Geometry: final body of the model. Coordinates: model frame, mm. A direction names the side the tool comes from. Give positions to 0.01 mm unless a question says otherwise; leave off trailing zeros. Write each loop counter-clockwise with the first axis right and the second up, starting at its lowest first coordinate (ties: lowest second). Pieces come first, ordered by that corner, then holes.
```python
from build123d import *

# Parameters (mm, degrees)
SKETCH1_R               = 8.25
BOSS_EXTRUDE1_DEPTH     = 135
BOSS_EXTRUDE2_DEPTH     = 2
CUT_EXTRUDE1_DEPTH      = 138.727992797
CUT_EXTRUDE1_DEPTH_BACK = 138.727992797
SKETCH4_R               = 1.6
SKETCH4_R_2             = 2.6
SKETCH4_R_3             = 3.727922061
SKETCH6_R               = 1.4
CUT_EXTRUDE2_DEPTH      = 140.11090078
CIRPATTERN1_COUNT       = 2
CIRPATTERN1_ANGLE       = 270
SKETCH7_R               = 6.269832862
CUT_EXTRUDE3_DEPTH      = 138.727992904


with BuildPart() as part:
    # Sketch1 → Boss-Extrude1 (new body)
    with BuildSketch(Plane.XY):
        Polygon((10, 4.142135624), (4.142135624, 10), (-4.142135624, 10), (-10, 4.142135624), (-10, -4.142135624), (-4.142135624, -10), (4.142135624, -10), (10, -4.142135624), align=None)
        Circle(SKETCH1_R, mode=Mode.SUBTRACT)
    extrude(amount=-BOSS_EXTRUDE1_DEPTH)

    # Sketch2 → Boss-Extrude2 (add)
    with BuildSketch(Plane(origin=(0, 0, -135), x_dir=(-1, 0, 0), z_dir=(0, 0, -1))):
        Polygon((-10, 4.142135624), (-10, -4.142135624), (-4.142135624, -10), (4.142135624, -10), (10, -4.142135624), (10, 4.142135624), (4.142135624, 10), (-4.142135624, 10), align=None)
    extrude(amount=BOSS_EXTRUDE2_DEPTH)

    # Sketch4 → Cut-Extrude1 (cut, two sides: drawn at the far end of the back side and taken through both)
    with BuildSketch(Plane(origin=(0, 0, 0), x_dir=(1, 0, 0), z_dir=(0, 1, 0)).offset(-CUT_EXTRUDE1_DEPTH_BACK)):
        with Locations(Location((0, 131.593089119, 0), (0, 0, 270))):
            Circle(SKETCH4_R)
        with Locations(Location((0, 106.593089119, 0), (0, 0, 270))):
            Circle(SKETCH4_R)
        with Locations(Location((0, 35, 0), (0, 0, 270))):
            Circle(SKETCH4_R_2)
        with Locations(Location((0, 119.093089119, 0), (0, 0, 270))):
            Circle(SKETCH4_R_3)
    extrude(amount=CUT_EXTRUDE1_DEPTH + CUT_EXTRUDE1_DEPTH_BACK, mode=Mode.SUBTRACT)

    # Sketch6 → Cut-Extrude2 (cut, through all)
    with BuildSketch(Plane(origin=(-7.071067812, 7.071067812, 0), x_dir=(0, 0, 1), z_dir=(-0.7071067811865476, 0.7071067811865476, 0))):
        with Locations(Location((-13, 0, 0), (0, 0, 270))):
            Circle(SKETCH6_R)
        with Locations(Location((-5, 0, 0), (0, 0, 270))):
            Circle(SKETCH6_R)
    cut_extrude2 = extrude(amount=-CUT_EXTRUDE2_DEPTH, mode=Mode.SUBTRACT)

    # CirPattern1: Cut-Extrude2 ×2 about axis
    cirpattern1_axis = Axis((0, 0, 6.85), (0, 0, -1))
    for i in range(1, CIRPATTERN1_COUNT):
        add(cut_extrude2.rotate(cirpattern1_axis, i * CIRPATTERN1_ANGLE / (CIRPATTERN1_COUNT - 1)), mode=Mode.SUBTRACT)

    # Sketch7 → Cut-Extrude3 (cut, through all)
    with BuildSketch(Plane(origin=(0, 0, -137), x_dir=(-1, 0, 0), z_dir=(0, 0, -1))):
        Circle(SKETCH7_R)
    extrude(amount=-CUT_EXTRUDE3_DEPTH, mode=Mode.SUBTRACT)


solid = part.part
```
Item 1: Section C-C, the plane x = 0. State how many separate pieces and enclosed holes the cut face has, plus the area to 3 significant figures.
Found:
separate pieces: 10
enclosed holes: 0
area: 421 mm2
Item 2: Section A-A, the plane y = 0. Return the cut outline in (x, z), plus the area to 3 significant figures.
Found:
outline: (-10, -137) - (-6.27, -137) - (-6.27, -135) - (-8.25, -135) - (-8.25, 0) - (-10, 0) - close; (6.27, -137) - (10, -137) - (10, 0) - (8.25, 0) - (8.25, -135) - (6.27, -135) - close
area: 487 mm2
Item 3: Pull-direction query (Y, two-part tool) for faces 3 (the face through (-7.11, 7.03, -67.54)), 4 (the face through (10, 0, -68)), 5 (the face through (6, -3, -135)); classes: +Y half, -Y half, draft (parallel to the pull), parting line (faces both ways), or undercut.
Found:
face 3: +Y half
face 4: draft
face 5: undercut
Item 4: Section B-B, the plane z = -35. Return the cut outline in (x, y), plus the area to 3 significant figures.
Found:
outline: (-10, -4.14) - (-4.14, -10) - (-2.6, -10) - (-2.6, -7.83) arc R8.25 cw to (-2.6, 7.83) - (-2.6, 10) - (-4.14, 10) - (-10, 4.14) - close; (2.6, -10) - (4.14, -10) - (10, -4.14) - (10, 4.14) - (4.14, 10) - (2.6, 10) - (2.6, 7.83) arc R8.25 cw to (2.6, -7.83) - close
area: 97.9 mm2
Item 5: Line query: L1, parallel to Z at x = 0, y = -9; L2, parallel to Y at x = 0, z = -28; L3, parallel to X at y = -0.5, z = -13. Output: solid intervals per line, ascending.
Found:
L1: z = -137 to -133.19, -129.99 to -122.82, -115.37 to -108.19, -104.99 to -37.6, -32.4 to 0
L2: y = -10 to -8.25, 8.25 to 10
L3: x = -10 to -8.23, 8.23 to 10
Item 6: Pin query (flat end, axial travel): pin 1 Ø6 at (x, z) = (-8, -96.5) entering from +Y; pin 2 Ø1.5 at (y, z) = (5, -66.5) entering from +X. Return the tip coordinate at first contact, or that it passes through.
Found:
pin 1: stops at y = 9.14
pin 2: stops at x = 9.89
Item 7: Section D-D, the plane z = -49. Return the cut outline in (x, y).
Found:
outline: (-10, -4.14) - (-4.14, -10) - (4.14, -10) - (10, -4.14) - (10, 4.14) - (4.14, 10) - (-4.14, 10) - (-10, 4.14) - close; hole circle Ø16.5 at (0, 0)
Item 8: Reachability of faces 1 (the face through (7.62, -3.16, -66.55)), 2 (the face through (0.164, 8.955, -122.817)) from +Z, -Z, +X, -X, +Y, -Y: full face, straight path, thin tool, end or side. Return the list, or none.
Found:
face 1: +Z
face 2: +Y, -Y
